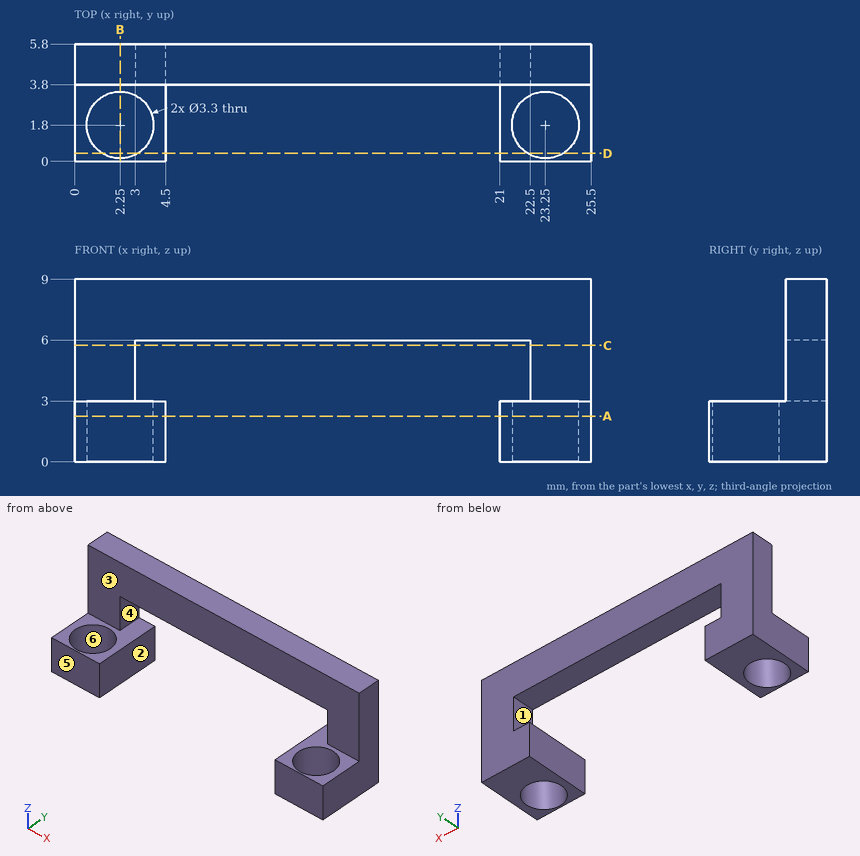
The drawing under review shows one solid part. Ordinate dimensions are in mm from its lowest x, y, z. A direction names the side the tool comes from. Coordinates: 2 decimals unless noted, no trailing zeros. Write each loop counter-clockwise with the first axis right and the second up, starting at its lowest first coordinate (ties: lowest second). Pieces come first, ordered by that corner, then holes.
1) Insertion check: pin 1 (1.3 mm diameter, centred on x = 22, y = 1.5, fed in from +Z); pin 2 (0.6 mm diameter, centred on x = 9.5, y = 5, fed in from -Z); pin 3 (1.8 mm diameter, centred on x = 9.5, z = 7, fed in from -Y); pin 4 (3 mm diameter, centred on x = 13.5, y = 2, fed in from +Z). Each pin has a flat end and moves straight along its axis. Give the tip position at first contact, or say it passes through.
2) To check wall thickness, follow L1, parallel to X at y = 1.8, z = 1.6; L2, parallel to X at y = 5.2, z = 4.25; L3, parallel to Y at x = 2.25, z = 1.45. State the ranges of each line that lie inside material, in increasing order.
3) Add section A-A (z = 2.25). Write out the cut boundary in (x, y).
4) Add section B-B (x = 2.25). Write out the cut boundary in (y, z).
5) Add section D-D (y = 0.4). Write out the cut boundary in (x, z).
6) Add section C-C (z = 5.75). Write out the cut boundary in (x, y), plus the area to 3 significant figures.
7) Machinability: for the marked faces 1, 2 and 3, which of the approach directions +Z, -Z, +X, -X, +Y, -Y give a long, thin tool a straight path to every point of the face, cutting with its end or side? Answer none if there is none.
8) Mouldability with a two-part tool opening along Y and no side actions: class the marked faces 4, 5 and 6 as +Y half, -Y half, draft (parallel to the pull), parting line (faces both ways), or undercut.
Check result:
1. pin 1: stops at z = 3
1. pin 2: stops at z = 6
1. pin 3: stops at y = 3.8
1. pin 4: passes through
2. L1: x = 0 to 0.6, 3.9 to 4.5, 21 to 21.6, 24.9 to 25.5
2. L2: x = 0 to 3, 22.5 to 25.5
2. L3: y = 0 to 0.15, 3.45 to 5.8
3. outline: (0, 0) - (4.5, 0) - (4.5, 5.8) - (0, 5.8) - close; (21, 0) - (25.5, 0) - (25.5, 5.8) - (21, 5.8) - close; hole circle Ø3.3 at (2.25, 1.8); hole circle Ø3.3 at (23.25, 1.8)
4. outline: (0, 0) - (0.15, 0) - (0.15, 3) - (0, 3) - close; (3.45, 0) - (5.8, 0) - (5.8, 9) - (3.8, 9) - (3.8, 3) - (3.45, 3) - close
5. outline: (0, 0) - (1.38, 0) - (1.38, 3) - (0, 3) - close; (3.12, 0) - (4.5, 0) - (4.5, 3) - (3.12, 3) - close; (21, 0) - (22.38, 0) - (22.38, 3) - (21, 3) - close; (24.12, 0) - (25.5, 0) - (25.5, 3) - (24.12, 3) - close
6. outline: (0, 3.8) - (3, 3.8) - (3, 5.8) - (0, 5.8) - close; (22.5, 3.8) - (25.5, 3.8) - (25.5, 5.8) - (22.5, 5.8) - close
6. area: 12.0 mm2
7. face 1: +Y, -Y
7. face 2: -Z, +Y, -Y
7. face 3: +Z, +X, -X, -Y
8. face 4: draft
8. face 5: -Y half
8. face 6: undercut
